Can you work these out from the model? Positions are in its coordinate system, mm. Round coordinates to 2 decimals unless told otherwise and drop trailing zeros. Write each loop counter-clockwise with the first axis right and the second up, starting at its lowest first coordinate (ties: lowest second). Pieces come first, ordered by that corner, then holes. Notation, with made-up numbers: M -12,52 L 15,52 A13 ccw 15,65 Z; hole C 28,-39 d2. An arc over 180 degrees is marked long. Answer in a Markdown table with one row per item. Add a question column.
(1) If we mould it in two halves opening along Y, with no side actions, what happens to faces 1 (the face through (-2.17, -9.76, 113.39)), 2 (the face through (-1.73, -7.81, 113.39)), 3 (the face through (0, 8.2, 0))? For each: released by +Y, released by -Y, zero draft, split by the parting line, or undercut.
(2) Suppose I cut it at C-C, the plane z = 56. Write out the boundary of the cut face in (x, y), then the cut area to 3 significant figures.
(3) If I drill on probe 1 along Y at (x, z) = (0.75, 117); probe 2 along Z at (x, y) = (-0.5, 8.5); probe 3 along X at (y, z) = (7.25, 37), over which ranges is the centre line in solid material (lowest first)?
(4) I'm going to push flat-ended pins straight in: pin 1 (5 mm diameter, centred on x = 2, y = -3.5, fed in from +Z); pin 2 (8 mm diameter, centred on y = -3, z = 205.5, fed in from -X); pin 3 (3 mm diameter, centred on y = -5.5, z = 162, fed in from +X); pin 4 (1 mm diameter, centred on x = 8, z = 204.5, fed in from +Y). Where does each tip first touch, or does it pass through?
(5) Suppose I cut it at B-B, the plane x = 4. Write out the boundary of the cut face in (y, z), then the cut area to 3 significant figures.
(6) Suppose I cut it at A-A, the plane y = 0. Write out the boundary of the cut face in (x, z), then the cut area to 3 significant figures.
from build123d import *

# Parameters (mm, degrees)
SKETCH_1_R               = 10
SKETCH_1_R_2             = 8
EXTRUDE_1_DEPTH          = 230
CUT_EXTRUDE_1_DEPTH      = 231.434372436
CUT_EXTRUDE_1_DEPTH_BACK = 230
SKETCH_2_R               = 1.55


with BuildPart() as part:
    # 草图1 → 凸台-拉伸1 (new body)
    with BuildSketch(Plane.XY):
        Circle(SKETCH_1_R)
        Circle(SKETCH_1_R_2, mode=Mode.SUBTRACT)
    extrude(amount=EXTRUDE_1_DEPTH)

    # 草图2 → 切除-拉伸1 (cut, two sides: drawn at the far end of the back side and taken through both)
    with BuildSketch(Plane(origin=(0, 0, 0), x_dir=(1, 0, 0), z_dir=(0, 1, 0)).offset(-CUT_EXTRUDE_1_DEPTH_BACK)):
        with Locations(Location((0, -10, 0), (0, 0, 90))):
            Circle(SKETCH_2_R)
        with Locations(Location((0, -25, 0), (0, 0, 90))):
            Circle(SKETCH_2_R)
        with Locations(Location((0, -220, 0), (0, 0, 90))):
            Circle(SKETCH_2_R)
        with Locations(Location((0, -205, 0), (0, 0, 90))):
            Circle(SKETCH_2_R)
    extrude(amount=CUT_EXTRUDE_1_DEPTH + CUT_EXTRUDE_1_DEPTH_BACK, mode=Mode.SUBTRACT)


solid = part.part
Calculated:
| question | item | result |
|---|---|---|
| 1 | face 1 | split by the parting line |
| 1 | face 2 | undercut |
| 1 | face 3 | zero draft |
| 2 | outline | C 0,0 d20; hole C 0,0 d16 |
| 2 | area | 113 mm² |
| 3 | probe 1 | -9.97 to -7.96, 7.96 to 9.97 |
| 3 | probe 2 | 0 to 8.53, 11.47 to 23.53, 26.47 to 203.53, 206.47 to 218.53, 221.47 to 230 |
| 3 | probe 3 | -6.89 to -3.38, 3.38 to 6.89 |
| 4 | pin 1 | through |
| 4 | pin 2 | x = -10 |
| 4 | pin 3 | x = 9.17 |
| 4 | pin 4 | y = 6.61 |
| 5 | outline | M -9.17,0 L -6.93,0 L -6.93,230 L -9.17,230 Z; M 6.93,0 L 9.17,0 L 9.17,230 L 6.93,230 Z |
| 5 | area | 1,030 mm² |
| 6 | outline | M -10,0 L -8,0 L -8,230 L -10,230 Z; M 8,0 L 10,0 L 10,230 L 8,230 Z |
| 6 | area | 920 mm² |
